CAD build for the part. Positions are in the model's coordinates, mm. Face numbers are marked on the shaded views. A direction names the side the tool comes from. Round coordinates to 2 decimals unless told otherwise and drop trailing zeros. Order: outer loops, then holes, each group sorted by start corner. A loop starts at its lowest first (then second) coordinate and runs counter-clockwise, first axis right, second up. Notation, with made-up numbers: (43.5, 9.5) -> (102.5, 9.5) arc R13 cw to (102.5, 17.5) -> close; hole circle Ø6 at (70.5, 45.25). An arc over 180 degrees is marked (long way). Return JSON: item names as keys, results as strings. Group by question number.
Q1. Mould opens along Y. For the marked faces 1, 2 and 3 say: +Y half, -Y half, draft (parallel to the pull), parting line (faces both ways), or undercut.
Q2. Cut at B-B (x = 22.65). Write the cut outline in (y, z).
Q3. Flat gauge pins, fed straight in: pin 1 (1.5 mm diameter, centred on x = 38.5, y = 15.5, fed in from -Z); pin 2 (1.5 mm diameter, centred on y = 4, z = -16.5, fed in from -X) (3 decimals); pin 3 (1 mm diameter, centred on y = 13, z = 1.5, fed in from -X). Where does each tip first touch, or does it go through?
Q4. Which spindle directions (+Z, -Z, +X, -X, +Y, -Y) get a long thin tool onto all of the face, cutting with end or side? Do the marked faces 4, 5 and 6. Say none if no direction does.
Q5. Cut at A-A (z = 0). Write the cut outline in (x, y).
Q6. Probe line 1 along Z through (x, y) = (0, 5); line 2 along X through (y, z) = (7.5, 0); line 3 along X through (y, z) = (17.55, 0). List the from-to ranges inside material, lowest first.
Q7. Cut at D-D (z = -22.65). Write the cut outline in (x, y), then the cut area to 3 significant figures.
Q8. Cut at C-C (y = 8). Write the cut outline in (x, z).
from build123d import *

# Parameters (mm, degrees)
SKETCH1_R                = 25.65
SKETCH1_R_2              = 19.65
SKETCH1_R_3              = 4
SKETCH1_R_4              = 0.95
SKETCH1_W                = 40.16
SKETCH1_H                = 20.39
BOSS_EXTRUDE2_DEPTH      = 3.7
SKETCH5_R                = 19.65
SKETCH5_W                = 40.16
SKETCH5_H                = 20.39
BOSS_EXTRUDE3_DEPTH      = 28.1
CUT_EXTRUDE1_REACH       = 133.143
SKETCH6_W                = 40.16
SKETCH6_H                = 28.1
CUT_EXTRUDE2_REACH       = 140.14
CUT_EXTRUDE2_END_RADIUS  = 25.65
SKETCH7_W                = 29.863740461
SKETCH7_H                = 10
CUT_EXTRUDE3_DEPTH       = 129.730214499
CUT_EXTRUDE3_DEPTH_BACK  = 129.730214499
SKETCH8_R                = 1.45
SKETCH9_R                = 0.95
CUT_EXTRUDE4_DEPTH       = 12
CUT_EXTRUDE5_DEPTH       = 129.730214499
FILLET1_R                = 2
CUT_EXTRUDE6_DEPTH       = 11.8
BOSS_EXTRUDE4_START      = -3.7
SKETCH14_R               = 19.65
SKETCH14_R_2             = 0.95
SKETCH14_R_3             = 4
BOSS_EXTRUDE4_DEPTH      = 3.7
CUT_EXTRUDE7_START       = -3.7
CUT_EXTRUDE7_OUTLINE_R   = 19.65
CUT_EXTRUDE7_OUTLINE_R_2 = 0.95
CUT_EXTRUDE7_OUTLINE_R_3 = 4
CUT_EXTRUDE7_DEPTH       = 3.7
SKETCH16_W               = 39.3
SKETCH16_H               = 31.8
CUT_EXTRUDE8_DEPTH       = 93.779590967


# Read off the part's stored shape, not the designer's step: Cut-Extrude7
with BuildPart() as part:
    # Sketch1 → Boss-Extrude2 (new body)
    # profile 1 of 6: a face of its own
    with BuildSketch(Plane(origin=(0, 0, 0), x_dir=(1, 0, 0), z_dir=(0, 1, 0))):
        Circle(SKETCH1_R)
        Circle(SKETCH1_R_2, mode=Mode.SUBTRACT)
    # profile 2 of 6: a face of its own
    with BuildSketch(Plane(origin=(0, 0, 0), x_dir=(1, 0, 0), z_dir=(0, 1, 0))):
        Circle(SKETCH1_R_2)
        with Locations(Location((0, 0, 0), (0, 0, 270))):
            Circle(SKETCH1_R_3, mode=Mode.SUBTRACT)
        with Locations(Location((16.6, 0, 0), (0, 0, 270))):
            Circle(SKETCH1_R_4, mode=Mode.SUBTRACT)
        with Locations(Location((0, -16.6, 0), (0, 0, 270))):
            Circle(SKETCH1_R_4, mode=Mode.SUBTRACT)
        with Locations(Location((-16.6, 0, 0), (0, 0, 270))):
            Circle(SKETCH1_R_4, mode=Mode.SUBTRACT)
        with Locations(Location((0, 16.6, 0), (0, 0, 270))):
            Circle(SKETCH1_R_4, mode=Mode.SUBTRACT)
    # profile 3 of 6: a face of its own
    with BuildSketch(Plane(origin=(0, 0, 0), x_dir=(1, 0, 0), z_dir=(0, 1, 0))):
        with BuildLine():
            Line((57.65, 18.695), (113.986875612, 18.695))
            ThreePointArc((113.986875612, 18.695), (105.869462663, 23.847948025), (96.425, 25.65))
            Line((96.425, 25.65), (0, 25.65))
            ThreePointArc((0, 25.65), (18.137288937, 18.137288937), (25.65, 0))
            ThreePointArc((25.65, 0), (18.137288937, -18.137288937), (0, -25.65))
            Line((0, -25.65), (96.425, -25.65))
            ThreePointArc((96.425, -25.65), (105.869462663, -23.847948025), (113.986875612, -18.695))
            Line((113.986875612, -18.695), (57.65, -18.695))
            Line((57.65, -18.695), (57.65, 18.695))
        make_face()
    # profile 4 of 6: a face of its own
    with BuildSketch(Plane(origin=(0, 0, 0), x_dir=(1, 0, 0), z_dir=(0, 1, 0))):
        with BuildLine():
            Line((114.81, -17.886147573), (114.81, 17.886147573))
            ThreePointArc((114.81, 17.886147573), (114.402987293, 18.295203548), (113.986875612, 18.695))
            Line((113.986875612, 18.695), (57.65, 18.695))
            Line((57.65, 18.695), (57.65, -18.695))
            Line((57.65, -18.695), (113.986875612, -18.695))
            ThreePointArc((113.986875612, -18.695), (114.402987293, -18.295203548), (114.81, -17.886147573))
        make_face()
        with Locations((86.23, 0)):
            Rectangle(SKETCH1_W, SKETCH1_H, mode=Mode.SUBTRACT)
    # profile 5 of 6: a face of its own
    with BuildSketch(Plane(origin=(0, 0, 0), x_dir=(1, 0, 0), z_dir=(0, 1, 0))):
        with Locations((86.23, 0)):
            Rectangle(SKETCH1_W, SKETCH1_H)
    # profile 6 of 6: a face of its own
    with BuildSketch(Plane(origin=(0, 0, 0), x_dir=(1, 0, 0), z_dir=(0, 1, 0))):
        with BuildLine():
            ThreePointArc((114.81, -17.886147573), (122.075, 0), (114.81, 17.886147573))
            Line((114.81, 17.886147573), (114.81, -17.886147573))
        make_face()
    extrude(amount=BOSS_EXTRUDE2_DEPTH)

    # Sketch5 → Boss-Extrude3 (add)
    # profile 1 of 4: a face of its own
    with BuildSketch(Plane(origin=(0, 3.7, 0), x_dir=(1, 0, 0), z_dir=(0, 1, 0))):
        with BuildLine():
            ThreePointArc((25.65, 0), (18.137288937, 18.137288937), (0, 25.65))
            ThreePointArc((0, 25.65), (-25.65, 0), (0, -25.65))
            ThreePointArc((0, -25.65), (18.137288937, -18.137288937), (25.65, 0))
        make_face()
        with Locations(Location((0, 0, 0), (0, 0, 270))):
            Circle(SKETCH5_R, mode=Mode.SUBTRACT)
    # profile 2 of 4: a face of its own
    with BuildSketch(Plane(origin=(0, 3.7, 0), x_dir=(1, 0, 0), z_dir=(0, 1, 0))):
        with BuildLine():
            ThreePointArc((114.81, 17.886147573), (114.402987293, 18.295203548), (113.986875612, 18.695))
            Line((113.986875612, 18.695), (57.65, 18.695))
            Line((57.65, 18.695), (57.65, -18.695))
            Line((57.65, -18.695), (113.986875612, -18.695))
            ThreePointArc((113.986875612, -18.695), (114.402987293, -18.295203548), (114.81, -17.886147573))
            Line((114.81, -17.886147573), (114.81, 17.886147573))
        make_face()
        with Locations((86.23, 0)):
            Rectangle(SKETCH5_W, SKETCH5_H, mode=Mode.SUBTRACT)
    # profile 3 of 4: a face of its own
    with BuildSketch(Plane(origin=(0, 3.7, 0), x_dir=(1, 0, 0), z_dir=(0, 1, 0))):
        with BuildLine():
            ThreePointArc((113.986875612, 18.695), (105.869462663, 23.847948025), (96.425, 25.65))
            Line((96.425, 25.65), (0, 25.65))
            ThreePointArc((0, 25.65), (18.137288937, 18.137288937), (25.65, 0))
            ThreePointArc((25.65, 0), (18.137288937, -18.137288937), (0, -25.65))
            Line((0, -25.65), (96.425, -25.65))
            ThreePointArc((96.425, -25.65), (105.869462663, -23.847948025), (113.986875612, -18.695))
            Line((113.986875612, -18.695), (57.65, -18.695))
            Line((57.65, -18.695), (57.65, 18.695))
            Line((57.65, 18.695), (113.986875612, 18.695))
        make_face()
    # profile 4 of 4: a face of its own
    with BuildSketch(Plane(origin=(0, 3.7, 0), x_dir=(1, 0, 0), z_dir=(0, 1, 0))):
        with BuildLine():
            ThreePointArc((114.81, -17.886147573), (122.075, 0), (114.81, 17.886147573))
            Line((114.81, 17.886147573), (114.81, -17.886147573))
        make_face()
    extrude(amount=BOSS_EXTRUDE3_DEPTH)

    # Sketch6 → Cut-Extrude1 (cut, up to next)
    with BuildSketch(Plane.XY.offset(-10.195), mode=Mode.PRIVATE) as cut_extrude1_sk1:
        with Locations((86.23, 17.75)):
            Rectangle(SKETCH6_W, SKETCH6_H)
    cut_extrude1_tool1 = extrude(cut_extrude1_sk1.sketch, amount=-CUT_EXTRUDE1_REACH, mode=Mode.PRIVATE) & part.part
    add(cut_extrude1_tool1.solids().sort_by_distance((86.23, 17.75, -10.195))[0], mode=Mode.SUBTRACT)

    # Cut-Extrude2: up to this cylinder (the profile starts inside it)
    cut_extrude2_end = Plane(origin=(96.425, 8.7, 0), z_dir=(0, -1, 0)) * Cylinder(CUT_EXTRUDE2_END_RADIUS, 332.58, mode=Mode.PRIVATE)
    # Sketch7 → Cut-Extrude2 (cut, up to the surface)
    with BuildSketch(Plane.ZY.offset(-106.31), mode=Mode.PRIVATE) as cut_extrude2_sk1:
        with Locations((-8.736870231, 8.7)):
            Rectangle(SKETCH7_W, SKETCH7_H)
    cut_extrude2_tool1 = extrude(cut_extrude2_sk1.sketch, amount=-CUT_EXTRUDE2_REACH, mode=Mode.PRIVATE) & cut_extrude2_end
    add(cut_extrude2_tool1.solids().sort_by_distance((106.31, 8.7, -8.73687))[0], mode=Mode.SUBTRACT)

    # Sketch8 → Cut-Extrude3 (cut, two sides: drawn at the far end of the back side and taken through both)
    with BuildSketch(Plane(origin=(0, 31.8, 0), x_dir=(1, 0, 0), z_dir=(0, 1, 0)).offset(-CUT_EXTRUDE3_DEPTH_BACK)):
        with Locations(Location((22.65, 0, 0), (0, 0, 270))):
            Circle(SKETCH8_R)
        with Locations(Location((0, -22.65, 0), (0, 0, 270))):
            Circle(SKETCH8_R)
        with Locations(Location((-22.65, 0, 0), (0, 0, 270))):
            Circle(SKETCH8_R)
        with Locations(Location((0, 22.65, 0), (0, 0, 270))):
            Circle(SKETCH8_R)
    extrude(amount=CUT_EXTRUDE3_DEPTH + CUT_EXTRUDE3_DEPTH_BACK, mode=Mode.SUBTRACT)

    # Sketch9 → Cut-Extrude4 (cut)
    with BuildSketch(Plane(origin=(0, 31.8, 0), x_dir=(1, 0, 0), z_dir=(0, 1, 0))):
        with Locations(Location((61.88, -4.95, 0), (0, 0, 270))):
            Circle(SKETCH9_R)
        with Locations(Location((61.88, 4.95, 0), (0, 0, 90))):
            Circle(SKETCH9_R)
        with Locations(Location((109.756875612, -4.95, 0), (0, 0, 90))):
            Circle(SKETCH9_R)
        with Locations(Location((109.756875612, 4.95, 0), (0, 0, 270))):
            Circle(SKETCH9_R)
    extrude(amount=-CUT_EXTRUDE4_DEPTH, mode=Mode.SUBTRACT)

    # Sketch12 → Cut-Extrude5 (cut, through all)
    with BuildSketch(Plane(origin=(0, 31.8, 0), x_dir=(1, 0, 0), z_dir=(0, 1, 0))):
        with BuildLine():
            Line((0, 25.65), (96.425, 25.65))
            ThreePointArc((96.425, 25.65), (105.19711491, 24.103371134), (112.911357997, 19.65))
            Line((112.911357997, 19.65), (16.486357997, 19.65))
            ThreePointArc((16.486357997, 19.65), (8.77211491, 24.103371134), (0, 25.65))
        make_face()
        with BuildLine():
            Line((0, -25.65), (96.425, -25.65))
            ThreePointArc((96.425, -25.65), (105.19711491, -24.103371134), (112.911357997, -19.65))
            Line((112.911357997, -19.65), (16.486357997, -19.65))
            ThreePointArc((16.486357997, -19.65), (8.77211491, -24.103371134), (0, -25.65))
        make_face()
    extrude(amount=-CUT_EXTRUDE5_DEPTH, mode=Mode.SUBTRACT)

    # Fillet1
    fillet1_edges = [part.edges().sort_by_distance(p)[0] for p in [
        (66.15, 17.75, -19.65),
        (106.31, 22.75, -19.65),
    ]]
    fillet(fillet1_edges, radius=FILLET1_R)

    # Sketch13 → Cut-Extrude6 (cut)
    with BuildSketch(Plane(origin=(0, 31.8, 0), x_dir=(1, 0, 0), z_dir=(0, 1, 0))):
        with BuildLine():
            Line((57.65, 19.65), (57.65, -19.65))
            Line((57.65, -19.65), (16.486357997, -19.65))
            ThreePointArc((16.486357997, -19.65), (-25.65, 0), (16.486357997, 19.65))
            Line((16.486357997, 19.65), (57.65, 19.65))
        make_face()
    extrude(amount=-CUT_EXTRUDE6_DEPTH, mode=Mode.SUBTRACT)

    # Sketch14 → Boss-Extrude4 (add)
    with BuildSketch(Plane(origin=(0, 20, 0), x_dir=(1, 0, 0), z_dir=(0, 1, 0)).offset(BOSS_EXTRUDE4_START)):
        with Locations(Location((0, 0, 0), (0, 0, 270))):
            Circle(SKETCH14_R)
        with Locations(Location((16.6, 0, 0), (0, 0, 270))):
            Circle(SKETCH14_R_2, mode=Mode.SUBTRACT)
        with Locations(Location((0, -16.6, 0), (0, 0, 270))):
            Circle(SKETCH14_R_2, mode=Mode.SUBTRACT)
        with Locations(Location((-16.6, 0, 0), (0, 0, 270))):
            Circle(SKETCH14_R_2, mode=Mode.SUBTRACT)
        with Locations(Location((0, 16.6, 0), (0, 0, 270))):
            Circle(SKETCH14_R_2, mode=Mode.SUBTRACT)
        with Locations(Location((0, 0, 0), (0, 0, 270))):
            Circle(SKETCH14_R_3, mode=Mode.SUBTRACT)
    extrude(amount=BOSS_EXTRUDE4_DEPTH)

    # Cut-Extrude7 outline → Cut-Extrude7 (cut)
    with BuildSketch(Plane.XZ.offset(CUT_EXTRUDE7_START)):
        Circle(CUT_EXTRUDE7_OUTLINE_R)
        with Locations((0, -16.6)):
            Circle(CUT_EXTRUDE7_OUTLINE_R_2, mode=Mode.SUBTRACT)
        with Locations((-16.6, 0)):
            Circle(CUT_EXTRUDE7_OUTLINE_R_2, mode=Mode.SUBTRACT)
        Circle(CUT_EXTRUDE7_OUTLINE_R_3, mode=Mode.SUBTRACT)
        with Locations((16.6, 0)):
            Circle(CUT_EXTRUDE7_OUTLINE_R_2, mode=Mode.SUBTRACT)
        with Locations((0, 16.6)):
            Circle(CUT_EXTRUDE7_OUTLINE_R_2, mode=Mode.SUBTRACT)
    extrude(amount=CUT_EXTRUDE7_DEPTH, mode=Mode.SUBTRACT)

    # Sketch16 → Cut-Extrude8 (cut, through all)
    with BuildSketch(Plane.ZY.offset(-57.65)):
        with Locations((0, 15.9)):
            Rectangle(SKETCH16_W, SKETCH16_H)
    extrude(amount=-CUT_EXTRUDE8_DEPTH, mode=Mode.SUBTRACT)


solid = part.part
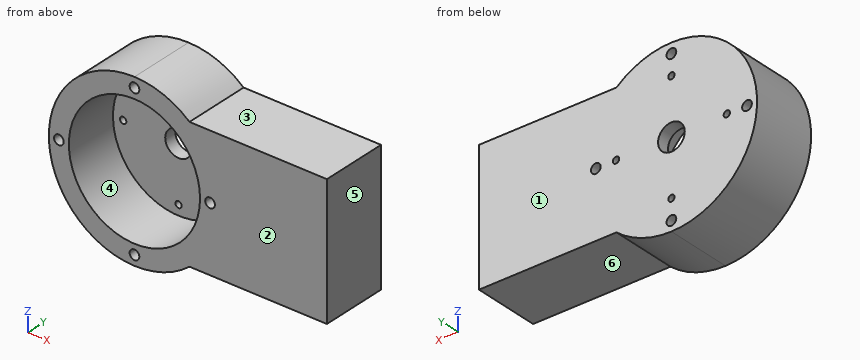
Solution:
{
 "1": {"face 1": "+Y half", "face 2": "-Y half", "face 3": "draft"},
 "2": {"outline": "(0, -19.65) -> (20, -19.65) -> (20, -1.45) -> (0, -1.45) -> close; (0, 1.45) -> (20, 1.45) -> (20, 19.65) -> (0, 19.65) -> close"},
 "3": {"pin 1": "stops at z = -19.65", "pin 2": "stops at x = -20.245", "pin 3": "stops at x = -25.63"},
 "4": {"face 4": "-Y", "face 5": "+Z, -Z, +X, +Y, -Y", "face 6": "-Z, +X, +Y, -Y"},
 "5": {"outline": "(-25.65, 0) -> (-24.1, 0) -> (-24.1, 20) -> (-25.65, 20) -> close; (-21.2, 0) -> (-19.65, 0) -> (-19.65, 16.3) -> (-17.55, 16.3) -> (-17.55, 20) -> (-21.2, 20) -> close; (-15.65, 16.3) -> (-4, 16.3) -> (-4, 20) -> (-15.65, 20) -> close; (4, 16.3) -> (15.65, 16.3) -> (15.65, 20) -> (4, 20) -> close; (17.55, 16.3) -> (19.65, 16.3) -> (19.65, 0) -> (21.2, 0) -> (21.2, 20) -> (17.55, 20) -> close; (24.1, 0) -> (57.65, 0) -> (57.65, 20) -> (24.1, 20) -> close"},
 "6": {"line 1": "z = -25.65 to -24.1, -21.2 to -19.65, 19.65 to 21.2, 24.1 to 25.65", "line 2": "x = -25.65 to -24.1, -21.2 to -19.65, 19.65 to 21.2, 24.1 to 57.65", "line 3": "x = -25.65 to -24.1, -21.2 to -17.55, -15.65 to -4, 4 to 15.65, 17.55 to 21.2, 24.1 to 57.65"},
 "7": {"outline": "(-12.04, 0) -> (-1.45, 0) -> (-1.45, 20) -> (-12.04, 20) -> close; (1.45, 0) -> (12.04, 0) -> (12.04, 20) -> (1.45, 20) -> close", "area": "423 mm²"},
 "8": {"outline": "(16.49, -19.65) -> (57.65, -19.65) -> (57.65, 19.65) -> (16.49, 19.65) arc R25.65 ccw (long way) to start; hole circle Ø2.9 at (-22.65, 0); hole circle Ø39.3 at (0, 0); hole circle Ø2.9 at (0, -22.65); hole circle Ø2.9 at (0, 22.65); hole circle Ø2.9 at (22.65, 0)"}
}
